Read the model definition and answer for the solid it produces. Units are mm, in the model's axes. Face numbers are marked on the shaded views. A direction names the side the tool comes from. Coordinates: 2 decimals unless noted, no trailing zeros. Order: outer loops, then holes, each group sorted by start corner. A loop starts at its lowest first (then second) coordinate and runs counter-clockwise, first axis right, second up. Notation, with made-up numbers: (-18.5, 50.25) - (2.5, 50.25) arc R11 ccw to (2.5, 54.25) - close; hole circle Ø3 at (87.25, -12.5). An arc over 180 degrees is marked (long way). Write item = value, one per line.
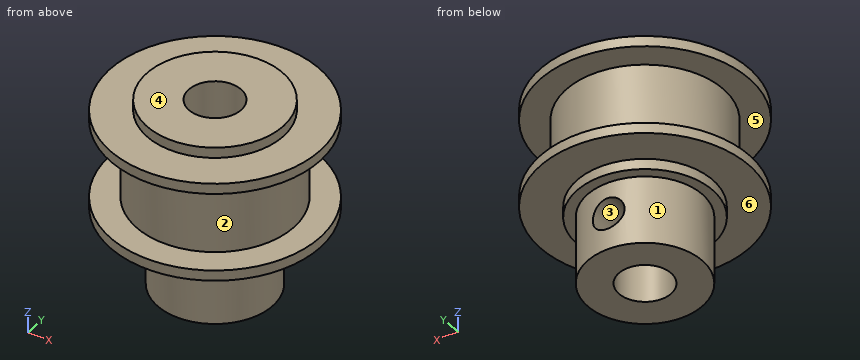
from build123d import *

# Parameters (mm, degrees)
SKETCH1_R                 = 5.5
BOSS_EXTRUDE1_DEPTH       = 6.5
SKETCH2_R                 = 6.5
BOSS_EXTRUDE2_DEPTH       = 1
SKETCH3_R                 = 10
BOSS_EXTRUDE3_DEPTH       = 1
SKETCH4_R                 = 7.51
BOSS_EXTRUDE4_DEPTH       = 7.5
SKETCH5_R                 = 10
BOSS_EXTRUDE5_DEPTH       = 1
SKETCH6_R                 = 6.5
BOSS_EXTRUDE6_DEPTH       = 1
SKETCH7_R                 = 2.5
CUT_EXTRUDE1_DEPTH        = 23.891046285
F_3_0MM_DOWEL_HOLE1_D     = 3
F_3_0MM_DOWEL_HOLE1_DEPTH = 5.5
F_3_0MM_DOWEL_HOLE1_TIP   = 0.901290929


with BuildPart() as part:
    # Sketch1 → Boss-Extrude1 (new body)
    with BuildSketch(Plane.XY):
        with Locations(Location((0, 0, 0), (0, 0, 180))):
            Circle(SKETCH1_R)
    extrude(amount=BOSS_EXTRUDE1_DEPTH)

    # Sketch2 → Boss-Extrude2 (add)
    with BuildSketch(Plane.XY.offset(6.5)):
        Circle(SKETCH2_R)
    extrude(amount=BOSS_EXTRUDE2_DEPTH)

    # Sketch3 → Boss-Extrude3 (add)
    with BuildSketch(Plane.XY.offset(7.5)):
        Circle(SKETCH3_R)
    extrude(amount=BOSS_EXTRUDE3_DEPTH)

    # Sketch4 → Boss-Extrude4 (add)
    with BuildSketch(Plane.XY.offset(8.5)):
        Circle(SKETCH4_R)
    extrude(amount=BOSS_EXTRUDE4_DEPTH)

    # Sketch5 → Boss-Extrude5 (add)
    with BuildSketch(Plane.XY.offset(16)):
        Circle(SKETCH5_R)
    extrude(amount=BOSS_EXTRUDE5_DEPTH)

    # Sketch6 → Boss-Extrude6 (add)
    with BuildSketch(Plane.XY.offset(17)):
        Circle(SKETCH6_R)
    extrude(amount=BOSS_EXTRUDE6_DEPTH)

    # Sketch7 → Cut-Extrude1 (cut, through all)
    with BuildSketch(Plane.XY.offset(18)):
        Circle(SKETCH7_R)
    extrude(amount=-CUT_EXTRUDE1_DEPTH, mode=Mode.SUBTRACT)

    # Ø3.0mm Dowel Hole1
    with Locations(Plane(origin=(0, 5.5, 3.5), x_dir=(1, 0, 0), z_dir=(0, 1, 0))):
        with Locations((0, 0)):
            Hole(F_3_0MM_DOWEL_HOLE1_D / 2, depth=F_3_0MM_DOWEL_HOLE1_DEPTH)
            with Locations((0, 0, -(F_3_0MM_DOWEL_HOLE1_DEPTH + F_3_0MM_DOWEL_HOLE1_TIP / 2))):  # 118° drill point
                Cone(0, F_3_0MM_DOWEL_HOLE1_D / 2, F_3_0MM_DOWEL_HOLE1_TIP, mode=Mode.SUBTRACT)


solid = part.part
1) The part is cut by section B-B (y = 0). Determine the outline of the cut face in (x, z).
Returned:
outline = (-10, 7.5) - (-6.5, 7.5) - (-6.5, 6.5) - (-5.5, 6.5) - (-5.5, 0) - (-2.5, 0) - (-2.5, 18) - (-6.5, 18) - (-6.5, 17) - (-10, 17) - (-10, 16) - (-7.51, 16) - (-7.51, 8.5) - (-10, 8.5) - close; (2.5, 0) - (5.5, 0) - (5.5, 6.5) - (6.5, 6.5) - (6.5, 7.5) - (10, 7.5) - (10, 8.5) - (7.51, 8.5) - (7.51, 16) - (10, 16) - (10, 17) - (6.5, 17) - (6.5, 18) - (2.5, 18) - close
2) The part is cut by section D-D (y = 6). Determine the outline of the cut face in (x, z), and give its area (3 significant figures).
Returned:
outline = (-8, 7.5) - (-2.5, 7.5) - (-2.5, 6.5) - (2.5, 6.5) - (2.5, 7.5) - (8, 7.5) - (8, 8.5) - (4.52, 8.5) - (4.52, 16) - (8, 16) - (8, 17) - (2.5, 17) - (2.5, 18) - (-2.5, 18) - (-2.5, 17) - (-8, 17) - (-8, 16) - (-4.52, 16) - (-4.52, 8.5) - (-8, 8.5) - close
area = 110 mm^2
3) Straight lines are drawn through the part: line 1 along Z through (x, y) = (0, 2.75); line 2 along Z through (x, y) = (6.5, -5); line 3 along Y through (x, z) = (0, 14). For each, find the intervals that lie inside material, in ascending order. Write a range as from..to.
Returned:
line_1 = 0..2, 5..18
line_2 = 7.5..8.5, 16..17
line_3 = -7.51..-2.5, 2.5..7.51
4) For the marked faces 1, 2 and 3, determine the directions among +Z, -Z, +X, -X, +Y, -Y from which every point of the face is accessible in a straight line to the end or side of a thin tool.
Returned:
face_1 = -Z
face_2 = none
face_3 = +Y
5) The part is cut by section C-C (z = 13). Determine the outline of the cut face in (x, y).
Returned:
outline = circle Ø15.02 at (0, 0); hole circle Ø5 at (0, 0)
6) The part is cut by section A-A (x = 0). Count the separate pieces of the cut face and the enclosed holes in it, and give its area (3 significant figures).
Returned:
separate_pieces = 3
enclosed_holes = 0
area = 151 mm^2
7) Flat-ended cylindrical pins translate along their axes: pin 1 Ø6 at (y, z) = (7.5, 4) entering from -X; pin 2 Ø3 at (y, z) = (-5, 15.5) entering from +X (3 decimals); pin 3 Ø2 at (y, z) = (-5.5, 10.5) entering from -X. Find the tip coordinate at first contact, or state that the pin passes through.
Returned:
pin_1 = -3.16
pin_2 = 9.335
pin_3 = -6.01
8) Determine the mould class of the marked faces 4, 5 and 6 for opening direction Z: pulls with the +Z half, pulls with the -Z half, needs draft (parallel to the pull), parting line crosses it, or undercut.
Returned:
face_4 = pulls with the +Z half
face_5 = undercut
face_6 = pulls with the -Z half
